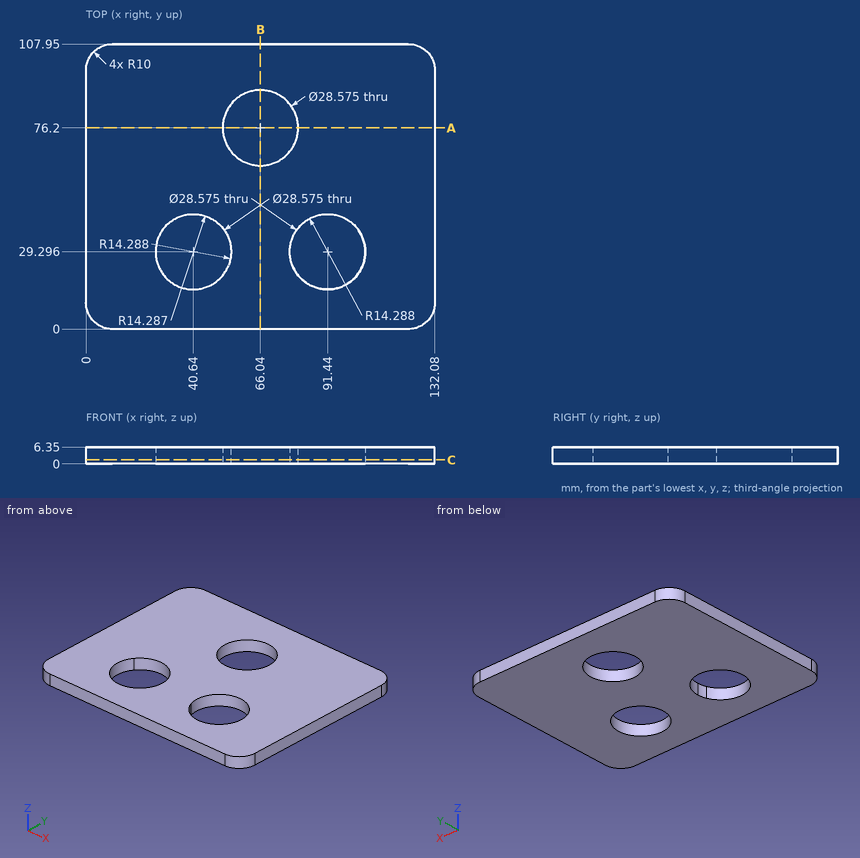
Job drawing, mm, ordinate dimensions from the low corner. One solid piece. Give positions to 0.01 mm unless a question says otherwise; leave off trailing zeros. Loops run counter-clockwise (first coordinate to the right, second up) from the corner with the lowest first, then second, coordinate; pieces in that order, holes last.
Item 1: Slice it at C-C, the plane z = 1.5. Give the number of separate pieces and of enclosed holes in the cut face, and give its area (3 significant figures).
Answers follow:
separate pieces: 1
enclosed holes: 3
area: 12,200 mm2
Item 2: Drill centre lines: line 1 (X direction, y = 76, z = 1); line 2 (Y direction, x = 66.04, z = 1.5); line 3 (Y direction, x = 40.64, z = 5). Where is each one in solid material? Low to high.
Answers follow:
line 1: x = 0 to 51.75, 80.33 to 132.08
line 2: y = 0 to 61.91, 90.49 to 107.95
line 3: y = 0 to 15.01, 43.58 to 107.95
Item 3: Slice it at A-A, the plane y = 76.2. List the corners of the cut face in (x, z), and give its area (3 significant figures).
Answers follow:
outline: (0, 0) - (51.75, 0) - (51.75, 6.35) - (0, 6.35) - close; (80.33, 0) - (132.08, 0) - (132.08, 6.35) - (80.33, 6.35) - close
area: 657 mm2
Item 4: Flat gauge pin, fed straight in: pin 1 (1 mm diameter, centred on y = 75.5, z = 1, fed in from -X). Where does the tip first touch, or does it go through?
Answers follow:
pin 1: stops at x = 0
Item 5: Slice it at B-B, the plane x = 66.04. List the corners of the cut face in (y, z).
Answers follow:
outline: (0, 0) - (61.91, 0) - (61.91, 6.35) - (0, 6.35) - close; (90.49, 0) - (107.95, 0) - (107.95, 6.35) - (90.49, 6.35) - close
